Check sheet for the drawn part. Datum: minimum x, y, z corner. Units: mm. A direction names the side the tool comes from. Coordinates: 2 decimals unless noted, no trailing zeros. Order: outer loops, then holes, each group sorted by start corner. A loop starts at its lowest first (then second) coordinate and runs counter-clockwise, first axis right, second up.
1. Cross-section at C-C (y = 25). Enter the section's corners in (x, z) (1 decimal), then the cut area to 3 significant figures.
2. Gauge pin test, flat ends, axial feed: pin 1 Ø5 at (y, z) = (8, 2.5) entering from -X; pin 2 Ø3 at (x, y) = (12, 16.5) entering from +Z; pin 3 Ø2 at (y, z) = (14, 3) entering from -X; pin 4 Ø4 at (x, z) = (10, 3) entering from +Y. Record the tip position at first contact, or that the pin passes through.
3. Draft check along X on the marked faces 1 and 2. Enter one of: released by +X, released by -X, zero draft, split by the parting line, or undercut.
4. Set-up check for the marked faces 3, 4 and 5: record each of +Z, -Z, +X, -X, +Y, -Y from which the full face is reachable in a straight line by a thin tool's end or side.
5. Thickness scan on line 1 (X direction, y = 20.5, z = 9) (1 decimal); line 2 (X direction, y = 29, z = 5.5) (1 decimal); line 3 (Y direction, x = 22, z = 8.5). Record the ranges inside material, lowest first.
6. Cross-section at B-B (x = 18.5). Enter the section's corners in (y, z) (1 decimal).
7. Cross-section at D-D (x = 24). Enter the section's corners in (y, z) (1 decimal), then the cut area to 3 significant figures.
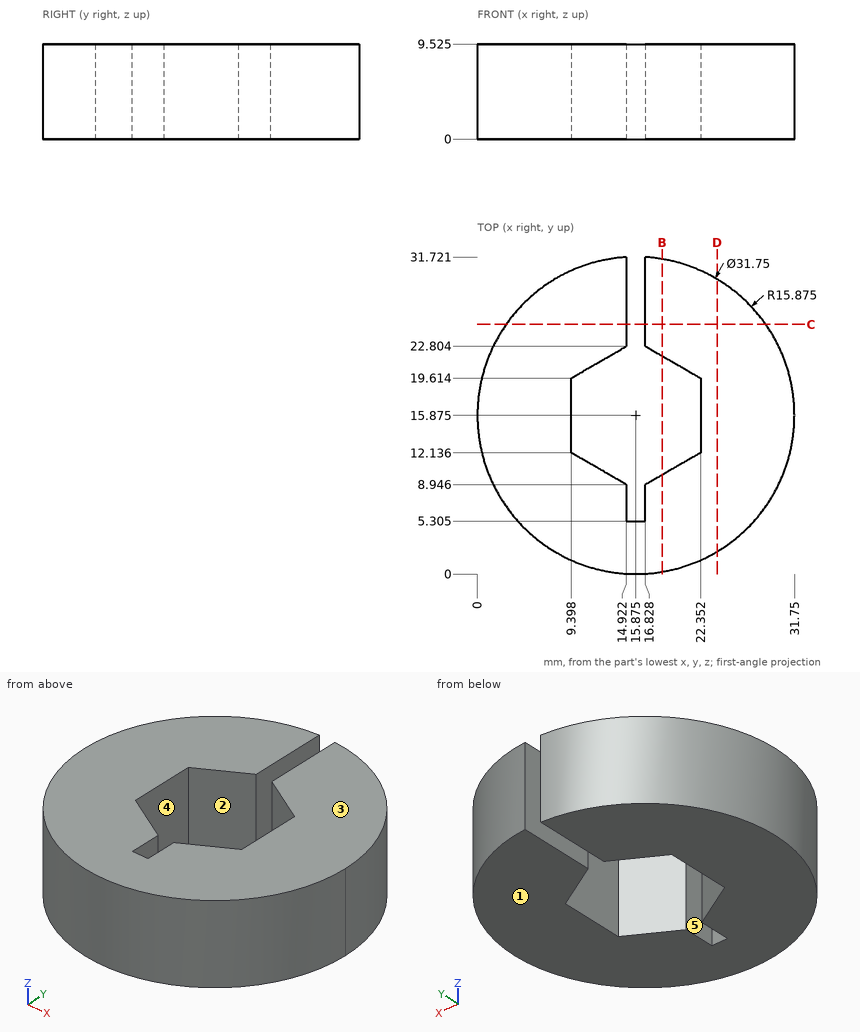
Data:
1. outline: (2.9, 0) - (14.9, 0) - (14.9, 9.5) - (2.9, 9.5) - close; (16.8, 0) - (28.9, 0) - (28.9, 9.5) - (16.8, 9.5) - close
1. area: 229 mm2
2. pin 1: stops at x = 0.94
2. pin 2: passes through
2. pin 3: stops at x = 0.02
2. pin 4: stops at y = 31.27
3. face 1: zero draft
3. face 2: undercut
4. face 3: +Z, +X, -X, +Y, -Y
4. face 4: +Z, -Z
4. face 5: +Z, -Z, +Y
5. line 1: x = 0.7 to 10.9, 20.8 to 31.1
5. line 2: x = 6.9 to 14.9, 16.8 to 24.8
5. line 3: y = 1.23 to 11.93, 19.82 to 30.52
6. outline: (0.2, 0) - (9.9, 0) - (9.9, 9.5) - (0.2, 9.5) - close; (21.8, 0) - (31.5, 0) - (31.5, 9.5) - (21.8, 9.5) - close
7. outline: (2.2, 0) - (29.5, 0) - (29.5, 9.5) - (2.2, 9.5) - close
7. area: 260 mm2
